Check sheet for the drawn part. Datum: minimum x, y, z corner. Units: mm. Give positions to 0.01 mm unless a question says otherwise; leave off trailing zeros. Write each loop counter-clockwise with the first axis right and the second up, starting at its lowest first coordinate (ties: lowest second). Pieces come first, ordered by that corner, then holes.
(1) Thickness scan on line 1 along Y through (x, z) = (87.5, 5.5); line 2 along X through (y, z) = (18, 6); line 3 along X through (y, z) = (3.75, 8.25). Record the ranges inside material, lowest first.
(2) Cross-section at C-C (y = 6). Record the boundary of the cut face in (x, z).
(3) Cross-section at A-A (x = 87.5). Record the boundary of the cut face in (y, z), and give its area (3 significant figures).
(4) Cross-section at B-B (z = 4.75). Record the boundary of the cut face in (x, y).
(5) Depth check by flat-ended pin: P1, Ø6, axis at y = 18, z = 5.5, coming from the -X side. Enter the tip coordinate at first touch or a pass-through.
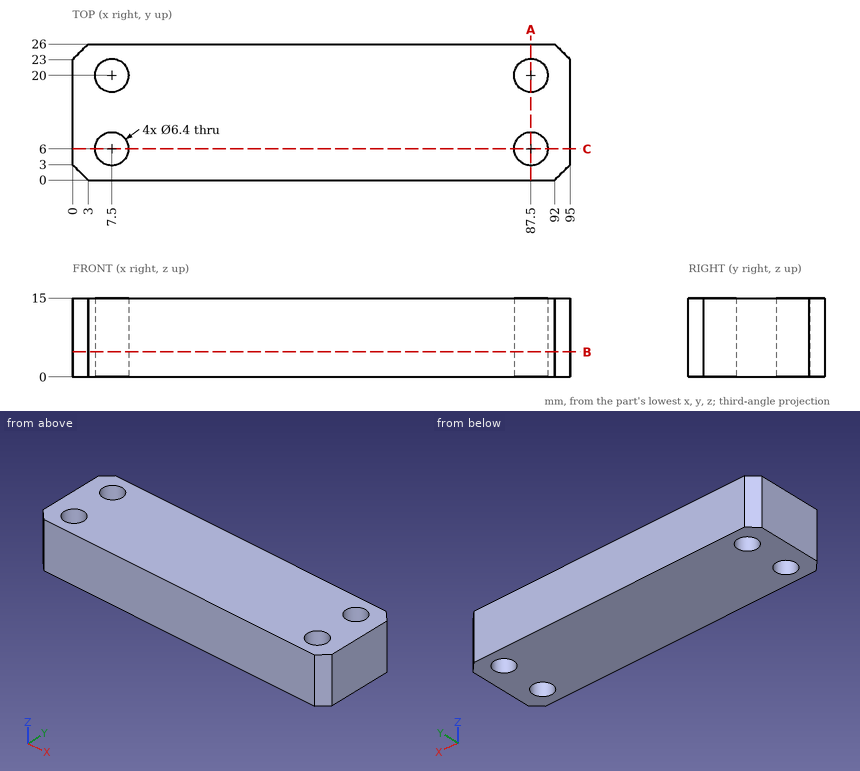
Reply:
1. line 1: y = 0 to 2.8, 9.2 to 16.8, 23.2 to 26
1. line 2: x = 0 to 5, 10 to 85, 90 to 95
1. line 3: x = 0 to 5.22, 9.78 to 85.22, 89.78 to 95
2. outline: (0, 0) - (4.3, 0) - (4.3, 15) - (0, 15) - close; (10.7, 0) - (84.3, 0) - (84.3, 15) - (10.7, 15) - close; (90.7, 0) - (95, 0) - (95, 15) - (90.7, 15) - close
3. outline: (0, 0) - (2.8, 0) - (2.8, 15) - (0, 15) - close; (9.2, 0) - (16.8, 0) - (16.8, 15) - (9.2, 15) - close; (23.2, 0) - (26, 0) - (26, 15) - (23.2, 15) - close
3. area: 198 mm2
4. outline: (0, 3) - (3, 0) - (92, 0) - (95, 3) - (95, 23) - (92, 26) - (3, 26) - (0, 23) - close; hole circle Ø6.4 at (7.5, 6); hole circle Ø6.4 at (7.5, 20); hole circle Ø6.4 at (87.5, 6); hole circle Ø6.4 at (87.5, 20)
5. P1: stops at x = 0
